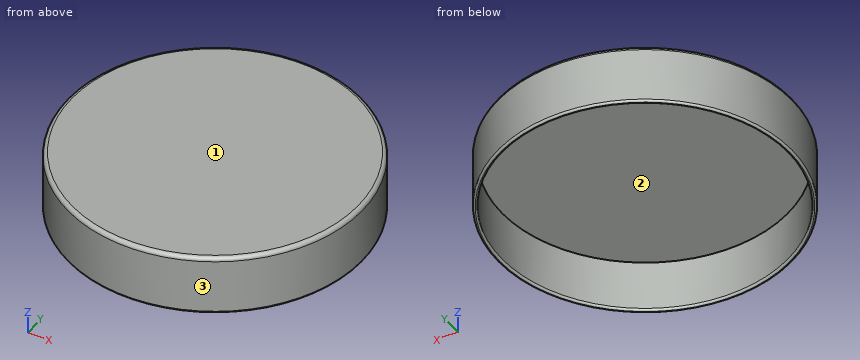
from build123d import *

# Parameters (mm, degrees)
F0_R     = 37
F0_R_2   = 36
F1_DEPTH = 15
F2_R     = 36.9218427358
F3_DEPTH = 2
F4_R     = 1
F5_R     = 0.49999


# Not quite as in the source:
# - a fillet or chamfer is up to 0.001 mm smaller than in the source, because OpenCascade refuses the exact size


with BuildPart() as f1:
    # F0 (on Top) → F1 (new body)
    with BuildSketch(Plane.XY):
        Circle(F0_R)
        Circle(F0_R_2, mode=Mode.SUBTRACT)
    extrude(amount=F1_DEPTH)

    # F2 (on face) → F3 (join)
    with BuildSketch(Plane.XY.offset(15)):
        Circle(F2_R)
    extrude(amount=-F3_DEPTH)

    # F4
    f4_edges = [f1.edges().sort_by_distance(p)[0] for p in [
        (-37, 0, 15),
    ]]
    fillet(f4_edges, radius=F4_R)

    # F5 (radius 0.5 in the source; OpenCascade refuses exactly that, so slightly less here)
    f5_edges = [f1.edges().sort_by_distance(p)[0] for p in [
        (-37, 0, 0),
        (-36, 0, 0),
    ]]
    fillet(f5_edges, radius=F5_R)


solid = f1.part
Design review of the part built by this model. Coordinates are the model's own, in mm. Face numbers are marked on the shaded views. Round coordinates to 2 decimals unless told otherwise and drop trailing zeros. Order: outer loops, then holes, each group sorted by start corner. A loop starts at its lowest first (then second) coordinate and runs counter-clockwise, first axis right, second up.
1) Draft analysis for pull direction Y (two halves, no side actions). For the marked faces 1, 2 and 3, state which applies: released by +Y, released by -Y, zero draft, split by the parting line, or undercut.
The answers:
face 1: zero draft
face 2: undercut
face 3: split by the parting line
2) Clearance check with flat-ended pins moving along their axes: pin 1 Ø8 at (x, y) = (2.5, 29.5) entering from -Z; pin 2 Ø6 at (y, z) = (-4, 12) entering from +X; pin 3 Ø4 at (y, z) = (29.5, 9) entering from -X. State where each tip first meets the part, or that it passes through.
The answers:
pin 1: stops at z = 13
pin 2: stops at x = 36.99
pin 3: stops at x = -24.75
3) For L1, parallel to Y at x = 0, z = 4.75; L2, parallel to Z at x = 19, y = -0.5; L3, parallel to X at y = -20, z = 6.25, list the stretches that pass through material, from the lowest coordinate up.
The answers:
L1: y = -37 to -36, 36 to 37
L2: z = 13 to 15
L3: x = -31.13 to -29.93, 29.93 to 31.13
4) Consider section C-C (z = 4.75). State the section outline as (x, y) points, plus the area to 3 significant figures.
The answers:
outline: circle Ø74 at (0, 0); hole circle Ø72 at (0, 0)
area: 229 mm2
